from build123d import *

# Parameters (mm, degrees)
F1_DEPTH = 20
F3_DEPTH = 25


with BuildPart() as f1:
    # F0 (on Front) → F1 (new body)
    with BuildSketch(Plane.XZ):
        Polygon((-32.5, -89.293016), (32.5, -89.293016), (82.292889, -47.511822), (93.58002, 16.500682), (61.08002, 72.792334), (0, 95.023643), (-61.08002, 72.792334), (-93.58002, 16.500682), (-82.292889, -47.511822), align=None)
    extrude(amount=F1_DEPTH)

    # F2 (on face) → F3 (cut)
    with BuildSketch(Plane.XZ.offset(20)):
        with BuildLine():
            Line((10, -42.5), (10, -36.142081))
            ThreePointArc((10, -36.142081), (0, 37.5), (-10, -36.142081))
            Line((-10, -36.142081), (-10, -42.5))
            Line((-10, -42.5), (0, -42.5))
            Line((0, -42.5), (10, -42.5))
        make_face()
    extrude(amount=-F3_DEPTH, mode=Mode.SUBTRACT)


solid = f1.part
The listing builds one solid part. Answer for the finished solid, in the listing's coordinates (mm). A direction names the side the tool comes from. Give positions to 0.01 mm unless a question says otherwise; leave off trailing zeros. Write each loop counter-clockwise with the first axis right and the second up, starting at its lowest first coordinate (ties: lowest second). Pieces come first, ordered by that corner, then holes.
Item 1: Section C-C, the plane z = 21.5 is taken. Write down the section's boundary in (x, y).
Item 2: Section D-D, the plane x = -58 is taken. Write down the section's boundary in (y, z).
Item 3: Which of the six approach directions +Z, -Z, +X, -X, +Y, -Y give full straight-line access (tool end or side, diameter ignored) to faces 1 (the flat face through (40, -20, 4)), 2 (the flat face through (10, -10, -39))?
Item 4: Section B-B, the plane z = 0 is taken. Write down the section's boundary in (x, y).
Item 5: Find the intervals of material crossed by line 1 along Z through (x, y) = (0, -8); line 2 along X through (y, z) = (-13.5, 0); line 3 along Z through (x, y) = (-8, -5.5), in increasing order.
Item 6: Flat-ended cylindrical pins translate along their axes: P1, Ø4, axis at y = -10.5, z = 55, coming from the +X side; P2, Ø1.9, axis at y = -9, z = -39.5, coming from the +X side; P3, Ø7, axis at y = -12, z = -38.5, coming from the -X side. Find the tip coordinate at first contact, or state that the pin passes through.
Item 7: Determine the mould class of faces 3 (the flat face through (0, -10, -42.5)), 4 (the flat face through (-88.015, -9.86, -15.057)), 5 (the flat face through (-77.103, -9.86, 45.041)), 6 (the flat face through (-10, -10, -39)) for opening direction Z: released by +Z, released by -Z, zero draft, split by the parting line, or undercut.
Item 8: Section A-A, the plane y = -5.75 is taken. Write down the section's boundary in (x, z).
Completed:
1. outline: (-90.69, -20) - (-30.72, -20) - (-30.72, 0) - (-90.69, 0) - close; (30.72, -20) - (90.69, -20) - (90.69, 0) - (30.72, 0) - close
2. outline: (-20, -67.9) - (0, -67.9) - (0, 73.91) - (-20, 73.91) - close
3. face 1: +Z, -Z, +X, -X, -Y
3. face 2: +Y, -Y
4. outline: (-90.67, -20) - (-37.5, -20) - (-37.5, 0) - (-90.67, 0) - close; (37.5, -20) - (90.67, -20) - (90.67, 0) - (37.5, 0) - close
5. line 1: z = -89.29 to -42.5, 37.5 to 95.02
5. line 2: x = -90.67 to -37.5, 37.5 to 90.67
5. line 3: z = -89.29 to -42.5, 36.64 to 92.11
6. P1: stops at x = 72.51
6. P2: stops at x = 83.87
6. P3: stops at x = -84.5
7. face 3: undercut
7. face 4: released by -Z
7. face 5: released by +Z
7. face 6: undercut
8. outline: (-93.58, 16.5) - (-82.29, -47.51) - (-32.5, -89.29) - (32.5, -89.29) - (82.29, -47.51) - (93.58, 16.5) - (61.08, 72.79) - (0, 95.02) - (-61.08, 72.79) - close; hole (-10, -42.5) - (10, -42.5) - (10, -36.14) arc R37.5 ccw (long way) to (-10, -36.14) - close
